Geometry check sheet. Reference: the model listing, model coordinates, mm. A direction names the side the tool comes from. Coordinates: 2 decimals unless noted, no trailing zeros. Loops run counter-clockwise (first coordinate to the right, second up) from the corner with the lowest first, then second, coordinate; pieces in that order, holes last. Notation, with made-up numbers: (76.5, 79) - (123.5, 79) arc R6 cw to (123.5, 88) - close; hole circle Ø10 at (-29, -11). An arc over 180 degrees is marked (long way). Write item = value, one per line. Start each with the question number.
from build123d import *

# Parameters (mm, degrees)
F0_W      = 1200
F0_H      = 720
F1_DEPTH  = 100
F2_T      = -3
F3_DEPTH  = 3
F4_R      = 20
F5_DEPTH  = 170
F6_W      = 840
F6_H      = 610
F7_DEPTH  = 85
F9_DEPTH  = 35
F11_DEPTH = 1200
F12_W     = 40
F12_H     = 800
F13_DEPTH = 2
F15_DEPTH = 38


with BuildPart() as f1:
    # F0 (on Top) → F1 (new body)
    with BuildSketch(Plane.XY):
        Rectangle(F0_W, F0_H)
    extrude(amount=F1_DEPTH)

    # F2
    f2_openings = [f1.faces().sort_by_distance(p)[0] for p in [
        (0, 0, 100),
    ]]
    offset(amount=F2_T, openings=f2_openings)

    # F3 (cut, through all): a face of the model
    f3_faces = [f1.faces().sort_by_distance(p)[0] for p in [
        (-597, 0, 51.5),
    ]]
    extrude(f3_faces, amount=-F3_DEPTH, mode=Mode.SUBTRACT)

    # F4 (on face) → F5 (join)
    with BuildSketch(Plane(origin=(0, 0, 0), x_dir=(1, 0, 0), z_dir=(0, 0, -1))):
        with Locations((-350, 250)):
            Circle(F4_R)
        with Locations((-350, 125)):
            Circle(F4_R)
        with Locations((-350, 0)):
            Circle(F4_R)
        with Locations((-350, -125)):
            Circle(F4_R)
        with Locations((-240, 250)):
            Circle(F4_R)
        with Locations((-240, 125)):
            Circle(F4_R)
        with Locations((-240, 0)):
            Circle(F4_R)
        with Locations((-240, -125)):
            Circle(F4_R)
        with Locations((-130, 250)):
            Circle(F4_R)
        with Locations((-130, 125)):
            Circle(F4_R)
        with Locations((-130, 0)):
            Circle(F4_R)
        with Locations((-130, -125)):
            Circle(F4_R)
        with Locations((-20, 250)):
            Circle(F4_R)
        with Locations((-20, 125)):
            Circle(F4_R)
        with Locations((-20, 0)):
            Circle(F4_R)
        with Locations((-20, -125)):
            Circle(F4_R)
        with Locations((90, 250)):
            Circle(F4_R)
        with Locations((90, 125)):
            Circle(F4_R)
        with Locations((90, 0)):
            Circle(F4_R)
        with Locations((90, -125)):
            Circle(F4_R)
        with Locations((200, 250)):
            Circle(F4_R)
        with Locations((200, 125)):
            Circle(F4_R)
        with Locations((200, 0)):
            Circle(F4_R)
        with Locations((200, -125)):
            Circle(F4_R)
        with Locations((310, 250)):
            Circle(F4_R)
        with Locations((310, 125)):
            Circle(F4_R)
        with Locations((310, 0)):
            Circle(F4_R)
        with Locations((310, -125)):
            Circle(F4_R)
        with Locations((-350, -250)):
            Circle(F4_R)
        with Locations((-240, -250)):
            Circle(F4_R)
        with Locations((-130, -250)):
            Circle(F4_R)
        with Locations((-20, -250)):
            Circle(F4_R)
        with Locations((90, -250)):
            Circle(F4_R)
        with Locations((200, -250)):
            Circle(F4_R)
        with Locations((310, -250)):
            Circle(F4_R)
    extrude(amount=F5_DEPTH)

    # F6 (on face) → F7 (join)
    with BuildSketch(Plane(origin=(0, 0, -170), x_dir=(1, 0, 0), z_dir=(0, 0, -1))):
        Rectangle(F6_W, F6_H)
    extrude(amount=F7_DEPTH)

    # F8 (on face) → F9 (join)
    with BuildSketch(Plane(origin=(0, 0, -255), x_dir=(1, 0, 0), z_dir=(0, 0, -1))):
        with BuildLine():
            Line((-300, 200), (-350, 200))
            ThreePointArc((-350, 200), (-400, 150), (-350, 100))
            Line((-350, 100), (-300, 100))
            ThreePointArc((-300, 100), (-250, 150), (-300, 200))
        make_face()
        with BuildLine():
            Line((250, 200), (200, 200))
            ThreePointArc((200, 200), (150, 150), (200, 100))
            Line((200, 100), (250, 100))
            ThreePointArc((250, 100), (300, 150), (250, 200))
        make_face()
        with BuildLine():
            Line((-300, -100), (-350, -100))
            ThreePointArc((-350, -100), (-400, -150), (-350, -200))
            Line((-350, -200), (-300, -200))
            ThreePointArc((-300, -200), (-250, -150), (-300, -100))
        make_face()
        with BuildLine():
            Line((250, -100), (200, -100))
            ThreePointArc((200, -100), (150, -150), (200, -200))
            Line((200, -200), (250, -200))
            ThreePointArc((250, -200), (300, -150), (250, -100))
        make_face()
    extrude(amount=F9_DEPTH)

    # F10 (on face) → F11 (join)
    with BuildSketch(Plane.YZ.offset(600)):
        Polygon((400, 100), (360, 100), (360, 98), (398, 98), (398, 60), (400, 60), align=None)
        Polygon((-360, 98), (-360, 100), (-400, 100), (-400, 60), (-398, 60), (-398, 98), align=None)
    extrude(amount=-F11_DEPTH)

    # F12 (on face) → F13 (join)
    with BuildSketch(Plane.XY.offset(100)):
        with Locations((620, 0)):
            Rectangle(F12_W, F12_H)
    extrude(amount=-F13_DEPTH)

    # F14 (on face) → F15 (join)
    with BuildSketch(Plane(origin=(0, 0, 98), x_dir=(1, 0, 0), z_dir=(0, 0, -1))):
        Polygon((638, -398), (600, -398), (600, -400), (640, -400), (640, 400), (600, 400), (600, 398), (638, 398), align=None)
    extrude(amount=F15_DEPTH)


solid = f1.part
(1) Sectioned sample at B-B on z = -133.5. Count the separate pieces of the cut face and the enclosed holes in it, plus the area to 3 significant figures.
(2) Tool access check on faces 1 (the face through (7, 357, 52)), 2 (the face through (-146, 137, -84)), 3 (the face through (-250.012, 151.099, -272.255)), 4 (the face through (-6, 305, -212)), 5 (the face through (-8, 360, 48)). Record the directions out of +Z, -Z, +X, -X, +Y, -Y that give a thin tool (end or side, any length) a straight path to the whole face; none if there is none.
(3) Scan lines: line 1 (X direction, y = -45.5, z = 76); line 2 (Z direction, x = 38.5, y = 155.5); line 3 (Y direction, x = 368.5, z = 14). Record each from-to range of solid material in increasing order.
(4) Depth check by flat-ended pin: pin 1 (3 mm diameter, centred on x = 381.5, y = 311, fed in from -Z); pin 2 (6 mm diameter, centred on x = 375, y = -176, fed in from -Z); pin 3 (10 mm diameter, centred on x = 15, y = -147, fed in from +Z); pin 4 (12 mm diameter, centred on y = -94, z = -86, fed in from -X). Enter the tip coordinate at first touch or a pass-through.
(5) Sectioned sample at A-A on y = -328. Enter the section's corners in (x, z), plus the area to 3 significant figures.
(6) Draft check along X on faces 6 (the face through (74, -113, -84)), 7 (the face through (299.988, 151.099, -272.255)), 8 (the face through (225, 200, -272)). Enter one of: pulls with the +X half, pulls with the -X half, needs draft (parallel to the pull), parting line crosses it, or undercut.
Working result:
q1.separate_pieces = 35
q1.enclosed_holes = 0
q1.area = 44,000 mm2
q2.face_1 = +Z, -X
q2.face_2 = none
q2.face_3 = -Z
q2.face_4 = -Z, +X, -X, +Y
q2.face_5 = -Z, -X
q3.line_1 = 597 to 600, 638 to 640
q3.line_2 = -255 to -170, 0 to 3
q3.line_3 = -360 to -357, 357 to 360
q4.pin_1 = 0
q4.pin_2 = -255
q4.pin_3 = 3
q4.pin_4 = through
q5.outline = (-600, 0) - (600, 0) - (600, 98) - (638, 98) - (638, 60) - (640, 60) - (640, 100) - (597, 100) - (597, 3) - (-600, 3) - close
q5.area = 4,050 mm2
q6.face_6 = undercut
q6.face_7 = pulls with the +X half
q6.face_8 = needs draft
